Part model, mm, in its own coordinate system. A direction names the side the tool comes from. Give positions to 0.01 mm unless a question says otherwise; leave off trailing zeros. Loops run counter-clockwise (first coordinate to the right, second up) from the corner with the lowest first, then second, coordinate; pieces in that order, holes last. Notation, with made-up numbers: M 19,24 L 32,24 A24 cw 32,46 Z; hole C 34.25,-10 d1. An arc over 180 degrees is marked long. Put each result on its own line as item: value. Start each with the question number.
```python
from build123d import *

# Parameters (mm, degrees)
F0_W     = 120
F0_H     = 100
F1_DEPTH = 50
F2_R     = 32.5
F3_DEPTH = 25
F5_DEPTH = 5


with BuildPart() as f1:
    # F0 (on Top) → F1 (new body)
    with BuildSketch(Plane.XY):
        Rectangle(F0_W, F0_H)
    extrude(amount=F1_DEPTH)

    # F2 (on face) → F3 (join)
    with BuildSketch(Plane.XY.offset(50)):
        Circle(F2_R)
    extrude(amount=F3_DEPTH)

    # F4 (on face) → F5 (join)
    with BuildSketch(Plane.XY.offset(75)):
        Polygon((-21.650635, -12.5), (0, -25), (21.650635, -12.5), (21.650635, 12.5), (0, 25), (-21.650635, 12.5), align=None)
    extrude(amount=F5_DEPTH)


solid = f1.part
```
1) Wall check: L1, parallel to Z at x = 6, y = -41; L2, parallel to Y at x = -2.5, z = 61.5; L3, parallel to X at y = -25, z = 57. Give the ranges that are in metal, low to high.
2) Pin check, flat tips, straight feed: pin 1 Ø4 at (x, z) = (-10.5, 61) entering from +Y; pin 2 Ø5 at (x, z) = (21, 59.5) entering from +Y; pin 3 Ø5.5 at (y, z) = (-4, 77) entering from -X. Stop position of each tip, or through.
3) Band-saw the part on D-D on y = 30. Give the cut face in (x, z).
4) Band-saw the part on A-A on y = 0. Give the cut face in (x, z), then the cut area to 3 significant figures.
5) Band-saw the part on B-B on x = -19. Give the cut face in (y, z), then the cut area to 3 significant figures.
6) Band-saw the part on C-C on z = 73.5. Give the cut face in (x, y).
7) Which spindle directions (+Z, -Z, +X, -X, +Y, -Y) get a long thin tool onto all of the face, cutting with end or side? Do faces 1 (the flat face through (10.67, -18.84, 77.46)), 2 (the flat face through (-1, 34, 50)), 3 (the flat face through (10.98, 18.66, 77.46)), 4 (the flat face through (-10.67, 18.84, 77.46)), 5 (the flat face through (21.651, 0, 77)). Say none if no direction does.
Evaluation:
1. L1: 0 to 50
1. L2: -32.4 to 32.4
1. L3: -20.77 to 20.77
2. pin 1: y = 31.37
2. pin 2: y = 26.72
2. pin 3: x = -32.43
3. outline: M -60,0 L 60,0 L 60,50 L 12.5,50 L 12.5,75 L -12.5,75 L -12.5,50 L -60,50 Z
4. outline: M -60,0 L 60,0 L 60,50 L 32.5,50 L 32.5,75 L 21.65,75 L 21.65,80 L -21.65,80 L -21.65,75 L -32.5,75 L -32.5,50 L -60,50 Z
4. area: 7,840 mm2
5. outline: M -50,0 L 50,0 L 50,50 L 26.37,50 L 26.37,75 L 14.03,75 L 14.03,80 L -14.03,80 L -14.03,75 L -26.37,75 L -26.37,50 L -50,50 Z
5. area: 6,460 mm2
6. outline: C 0,0 d65
7. face 1: +Z, +X, -Y
7. face 2: +Z
7. face 3: +Z, +X, +Y
7. face 4: +Z, -X, +Y
7. face 5: +Z, +X, +Y, -Y
